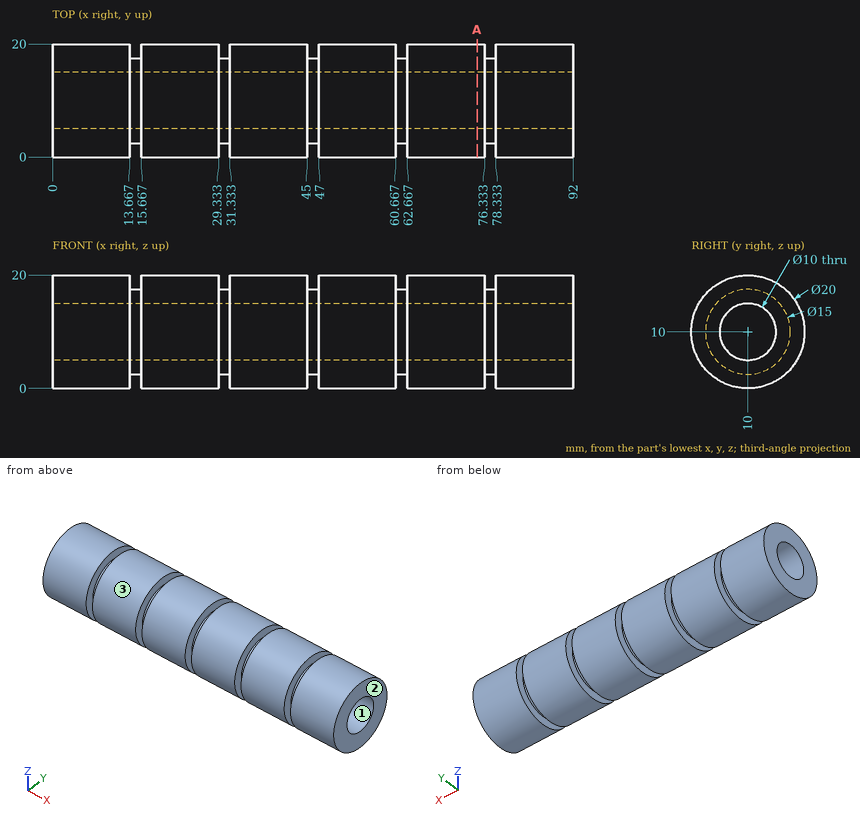
Part print with two shaded views. Sizes in mm from the minimum x, y, z corner. Coordinates: 2 decimals unless noted, no trailing zeros. Order: outer loops, then holes, each group sorted by start corner. A loop starts at its lowest first (then second) coordinate and runs counter-clockwise, first axis right, second up. Notation, with made-up numbers: (73, 1) - (89, 1) arc R20 ccw to (89, 20) - close; hole circle Ø11 at (69, 28). An arc over 180 degrees is marked (long way). Answer in a Markdown table with one row per item.
1. Drill centre lines: L1, parallel to X at y = 3, z = 14.75; L2, parallel to Y at x = 34, z = 10; L3, parallel to Y at x = 65.5, z = 13.5. Where is each one in solid material? Low to high. Write a range as from..to.
Answer:
| item | result |
|---|---|
| L1 | 0..13.67, 15.67..29.33, 31.33..45, 47..60.67, 62.67..76.33, 78.33..92 |
| L2 | 0..5, 15..20 |
| L3 | 0.63..6.43, 13.57..19.37 |
2. Flat gauge pins, fed straight in: P1, Ø10, axis at y = 7.5, z = 6, coming from the +X side; P2, Ø1.5, axis at x = 37, y = 17, coming from the +Z side; P3, Ø4, axis at x = 30, z = 12, coming from the -Y side. Where does each tip first touch, or does it go through?
Answer:
| item | result |
|---|---|
| P1 | x = 92 |
| P2 | z = 17.81 |
| P3 | y = 0 |
3. Pull direction Z, two halves, no side cores. Call the marked faces 1, 2 and 3: +Z half, -Z half, draft (parallel to the pull), parting line (faces both ways), or undercut.
Answer:
| item | result |
|---|---|
| face 1 | undercut |
| face 2 | draft |
| face 3 | parting line |
4. Slice it at A-A, the plane x = 75. List the corners of the cut face in (y, z).
Answer:
| item | result |
|---|---|
| outline | circle Ø20 at (10, 10); hole circle Ø10 at (10, 10) |
